```python
from build123d import *

# Parameters (mm, degrees)
BOX055_W          = 12
BOX055_H          = 4
BOX055_DEPTH      = 1.2
CYLINDER113_R     = 1.25
CYLINDER113_DEPTH = 10
CYLINDER112_R     = 1.25
CYLINDER112_DEPTH = 10
BOX048_W          = 16
BOX048_H          = 8.5
BOX048_DEPTH      = 17
FILLET024_R       = 2


with BuildPart() as cube034:
    # Box055 → Box055 (new body)
    with BuildSketch(Plane(origin=(325.5, 7.5, 9.4), x_dir=(1, 0, 0), z_dir=(0, 0, 1))):
        with Locations((6, 2)):
            Rectangle(BOX055_W, BOX055_H)
    extrude(amount=BOX055_DEPTH)


with BuildPart() as cylinder113:
    # Cylinder113 → Cylinder113 (new body)
    with BuildSketch(Plane(origin=(320, 26, 0), x_dir=(1, 0, 0), z_dir=(0, -1, 0))):
        Circle(CYLINDER113_R)
    extrude(amount=CYLINDER113_DEPTH)


with BuildPart() as fusion098:
    # Cylinder112 → Cylinder112 (new body)
    with BuildSketch(Plane(origin=(320, 26, 10), x_dir=(1, 0, 0), z_dir=(0, -1, 0))):
        Circle(CYLINDER112_R)
    extrude(amount=CYLINDER112_DEPTH)

    # Fusion098: union Cylinder113
    add(cylinder113.part)


with BuildPart() as fusion098_1:
    # Fusion098 placement: moved
    add(fusion098.part.moved(Location((16.5, -9.5, 4.5))))


with BuildPart() as cut062:
    # Box048 → Box048 (new body)
    with BuildSketch(Plane(origin=(323.5, 7.5, 1.5), x_dir=(1, 0, 0), z_dir=(0, 0, 1))):
        with Locations((8, 4.25)):
            Rectangle(BOX048_W, BOX048_H)
    extrude(amount=BOX048_DEPTH)

    # Cut059: cut Fusion098
    add(fusion098_1.part, mode=Mode.SUBTRACT)

    # Fillet024
    fillet024_edges = [cut062.edges().sort_by_distance(p)[0] for p in [
        (331.5, 7.5, 1.5),
        (331.5, 7.5, 18.5),
    ]]
    fillet(fillet024_edges, radius=FILLET024_R)

    # Cut062: cut Cube034
    add(cube034.part, mode=Mode.SUBTRACT)


with BuildPart() as cut062_1:
    # Cut062 placement: moved
    add(cut062.part.moved(Location((0, -16, 0))))


solid = cut062_1.part
```
Source: CAD feature listing. Evaluate the final solid. Frame: model axes, mm. A direction names the side the tool comes from. Round coordinates to 2 decimals unless told otherwise and drop trailing zeros. Order: outer loops, then holes, each group sorted by start corner. A loop starts at its lowest first (then second) coordinate and runs counter-clockwise, first axis right, second up. Notation, with made-up numbers: (-26, -9.5) -> (-7, -9.5) arc R26 cw to (-7, 27.5) -> close; hole circle Ø4 at (82, -36). An arc over 180 degrees is marked (long way). One line per item, written item: value. Start each with the question number.
Q1. Section query B-B (x = 335.5). Return the cut outline in (y, z), plus the area to 3 significant figures.
Q2. Pin query (flat end, axial travel): pin 1 (2 mm diameter, centred on x = 336.5, z = 4.5, fed in from -Y). Return the tip coordinate at first contact, or that it passes through.
Q3. Access query for faces 5 (the cylindrical face through (329.71, -7.93, 2.1)), 6 (the flat face through (331, 0, 10)), 7 (the flat face through (331, -4.5, 10)). Directions: +Z, -Z, +X, -X, +Y, -Y. A direction counts if a zero-diameter tool reaches every point of the face in a straight line with its end or side. Return the directions, or none.
Q4. Section query D-D (x = 333). Return the cut outline in (y, z).
Q5. Material intervals for probe 1 along Z at (x, y) = (336.5, -6); probe 2 along Z at (x, y) = (336.5, -3.25); probe 3 along Z at (x, y) = (333.75, -6.25), sorted ascending.
Q6. Draft query along X for faces 1 (the flat face through (323.5, -4, 10)), 2 (the cylindrical face through (331.61, -7.93, 17.9)), 3 (the flat face through (325.5, -7, 10)), 4 (the flat face through (331, -6, 9.4)). Return one class per face: pulls with the +X half, pulls with the -X half, needs draft (parallel to the pull), parting line crosses it, or undercut.
Q7. Section query A-A (z = 14.5). Return the cut outline in (x, y), plus the area to 3 significant figures.
Q8. Section query C-C (y = -3.75). Return the cut outline in (x, z), plus the area to 3 significant figures.
Findings below:
1. outline: (-8.5, 3.5) arc R2 ccw to (-6.5, 1.5) -> (0, 1.5) -> (0, 3.75) -> (-8.5, 3.75) -> close; (-8.5, 5.25) -> (0, 5.25) -> (0, 13.75) -> (-8.5, 13.75) -> (-8.5, 10.6) -> (-4.5, 10.6) -> (-4.5, 9.4) -> (-8.5, 9.4) -> close; (-8.5, 15.25) -> (0, 15.25) -> (0, 18.5) -> (-6.5, 18.5) arc R2 ccw to (-8.5, 16.5) -> close
1. area: 112 mm²
2. pin 1: through
3. face 5: -Z, -X, -Y
3. face 6: +Z, -Z, +X, -X, +Y
3. face 7: -Y
4. outline: (-8.5, 3.5) arc R2 ccw to (-6.5, 1.5) -> (0, 1.5) -> (0, 18.5) -> (-6.5, 18.5) arc R2 ccw to (-8.5, 16.5) -> (-8.5, 10.6) -> (-4.5, 10.6) -> (-4.5, 9.4) -> (-8.5, 9.4) -> close
5. probe 1: 1.5 to 3.25, 5.75 to 9.4, 10.6 to 13.25, 15.75 to 18.5
5. probe 2: 1.5 to 3.25, 5.75 to 13.25, 15.75 to 18.5
5. probe 3: 1.5 to 9.4, 10.6 to 18.5
6. face 1: pulls with the -X half
6. face 2: needs draft
6. face 3: undercut
6. face 4: undercut
7. outline: (323.5, -8.5) -> (335.25, -8.5) -> (335.25, 0) -> (323.5, 0) -> close; (337.75, -8.5) -> (339.5, -8.5) -> (339.5, 0) -> (337.75, 0) -> close
7. area: 115 mm²
8. outline: (323.5, 1.5) -> (339.5, 1.5) -> (339.5, 18.5) -> (323.5, 18.5) -> close; hole circle Ø2.5 at (336.5, 4.5); hole circle Ø2.5 at (336.5, 14.5)
8. area: 262 mm²
